Verification items for the finished model (mm, model axes). Face numbers are marked on the shaded views. A direction names the side the tool comes from. Round coordinates to 2 decimals unless told otherwise and drop trailing zeros. Order: outer loops, then holes, each group sorted by start corner. A loop starts at its lowest first (then second) coordinate and runs counter-clockwise, first axis right, second up. Notation, with made-up numbers: (9, 64) -> (29, 64) arc R16 cw to (29, 79) -> close; hole circle Ø2 at (81, -17.75). An arc over 180 degrees is marked (long way). Put each result on its own line as item: value.
from build123d import *

# Parameters (mm, degrees)
SKETCH1_W           = 46
SKETCH1_H           = 26
SKETCH1_W_2         = 40
SKETCH1_H_2         = 20
EXTRUDE_THIN1_DEPTH = 120
FILLET2_R           = 5


with BuildPart() as part:
    # Sketch1 → Extrude-Thin1 (new body)
    with BuildSketch(Plane.XY):
        Rectangle(SKETCH1_W, SKETCH1_H)
        Rectangle(SKETCH1_W_2, SKETCH1_H_2, mode=Mode.SUBTRACT)
    extrude(amount=EXTRUDE_THIN1_DEPTH)

    # Fillet2
    fillet2_edges = [part.edges().sort_by_distance(p)[0] for p in [
        (-23, 13, 60),
        (23, 13, 60),
        (23, -13, 60),
        (-23, -13, 60),
    ]]
    fillet(fillet2_edges, radius=FILLET2_R)


solid = part.part
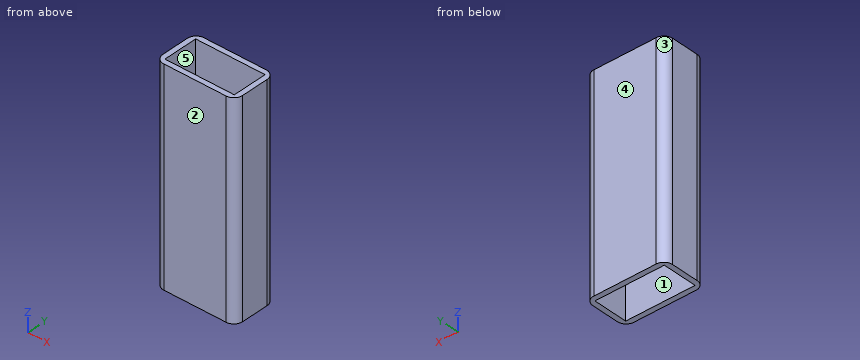
Item 1: Section check B-B on x = 8.5. Record the boundary of the cut face in (y, z), then the cut area to 3 significant figures.
Check sheet entries:
outline: (-13, 0) -> (-10, 0) -> (-10, 120) -> (-13, 120) -> close; (10, 0) -> (13, 0) -> (13, 120) -> (10, 120) -> close
area: 720 mm^2
Item 2: Tool access check on the marked faces 4 and 5. Record the directions out of +Z, -Z, +X, -X, +Y, -Y that give a thin tool (end or side, any length) a straight path to the whole face; none if there is none.
Check sheet entries:
face 4: +Z, -Z, +X, -X, +Y
face 5: +Z, -Z
Item 3: Gauge pin test, flat end, axial feed: pin 1 Ø1.5 at (x, y) = (18, 7.5) entering from -Z. Record the tip position at first contact, or that the pin passes through.
Check sheet entries:
pin 1: passes through
Item 4: Section check C-C on z = 93. Record the boundary of the cut face in (x, y).
Check sheet entries:
outline: (-23, -8) arc R5 ccw to (-18, -13) -> (18, -13) arc R5 ccw to (23, -8) -> (23, 8) arc R5 ccw to (18, 13) -> (-18, 13) arc R5 ccw to (-23, 8) -> close; hole (-20, -10) -> (20, -10) -> (20, 10) -> (-20, 10) -> close
Item 5: Section check A-A on y = -3.75. Record the boundary of the cut face in (x, z), then the cut area to 3 significant figures.
Check sheet entries:
outline: (-23, 0) -> (-20, 0) -> (-20, 120) -> (-23, 120) -> close; (20, 0) -> (23, 0) -> (23, 120) -> (20, 120) -> close
area: 720 mm^2
Item 6: Material ranges on L1, parallel to Y at x = 7.5, z = 83.5; L2, parallel to X at y = 6, z = 66.5; L3, parallel to X at y = 8.75, z = 58, recorded low to high. Write a range as [from, to].
Check sheet entries:
L1: y = [-13, -10], [10, 13]
L2: x = [-23, -20], [20, 23]
L3: x = [-22.94, -20], [20, 22.94]
Item 7: Release check for a two-part mould opening along Y. For the marked faces 1, 2 and 3 record: +Y half, -Y half, draft (parallel to the pull), parting line (faces both ways), or undercut.
Check sheet entries:
face 1: undercut
face 2: -Y half
face 3: +Y half
